The model under review builds one solid part; all positions refer to its coordinate system, in mm. A direction names the side the tool comes from. Coordinates: 2 decimals unless noted, no trailing zeros. Write each loop counter-clockwise with the first axis right and the second up, starting at its lowest first coordinate (ties: lowest second). Pieces come first, ordered by that corner, then holes.
```python
from build123d import *

# Parameters (mm, degrees)
F1_DEPTH = 24
F2_DEPTH = 12


with BuildPart() as f1:
    # F0 (on Front) → F1 (new body)
    with BuildSketch(Plane.XZ):
        Polygon((0, 32), (0, 0), (28.475209, 0), (10, 32), align=None)
        Polygon((10, 32), (28.475209, 0), (39.524791, 0), (58, 32), align=None)
        Polygon((58, 32), (39.524791, 0), (68, 0), (68, 32), align=None)
    extrude(amount=-F1_DEPTH)

    # F0 (on Front) → F2 (cut)
    with BuildSketch(Plane.XZ):
        Polygon((10, 32), (28.475209, 0), (39.524791, 0), (58, 32), align=None)
    extrude(amount=-F2_DEPTH, mode=Mode.SUBTRACT)


solid = f1.part
```
Item 1: Take a section at B-B, the plane z = 13.5. Write out the cut boundary in (x, y).
Solved:
outline: (0, 0) - (20.68, 0) - (20.68, 12) - (47.32, 12) - (47.32, 0) - (68, 0) - (68, 24) - (0, 24) - close
Item 2: For pin 1 (1 mm diameter, centred on x = 29.5, y = 6.5, fed in from +Z); pin 2 (6 mm diameter, centred on x = 16, y = 5.5, fed in from +Z), all flat-tipped, find the tip position at first contact; note any pin that passes through.
Solved:
pin 1: passes through
pin 2: stops at z = 26.8
Item 3: Take a section at A-A, the plane y = 7. Write out the cut boundary in (x, z).
Solved:
outline: (0, 0) - (28.48, 0) - (10, 32) - (0, 32) - close; (39.52, 0) - (68, 0) - (68, 32) - (58, 32) - close
Item 4: Machinability: for faces 5 (the face through (34, 14, 0)), 6 (the face through (34, 12, 20)), which of the approach directions +Z, -Z, +X, -X, +Y, -Y give a long, thin tool a straight path to every point of the face, cutting with its end or side? Answer none if there is none.
Solved:
face 5: -Z, +X, -X, +Y, -Y
face 6: +Z, -Y
Item 5: Take a section at D-D, the plane z = 7.5. Write out the cut boundary in (x, y).
Solved:
outline: (0, 0) - (24.15, 0) - (24.15, 12) - (43.85, 12) - (43.85, 0) - (68, 0) - (68, 24) - (0, 24) - close
Item 6: Mouldability with a two-part tool opening along X and no side actions: class faces 1 (the face through (19.11, 5.92, 16.22)), 2 (the face through (0, 12, 16)), 3 (the face through (34, 17, 32)), 4 (the face through (48.633, 5.916, 15.776)) as pulls with the +X half, pulls with the -X half, needs draft (parallel to the pull), parting line crosses it, or undercut.
Solved:
face 1: undercut
face 2: pulls with the -X half
face 3: needs draft
face 4: undercut
Item 7: To check wall thickness, follow line 1 along X through (y, z) = (8, 11.5); line 2 along X through (y, z) = (1.75, 16); line 3 along Z through (x, y) = (23, 3). State the ranges of each line that lie inside material, in increasing order.
Solved:
line 1: x = 0 to 21.84, 46.16 to 68
line 2: x = 0 to 19.24, 48.76 to 68
line 3: z = 0 to 9.48
Item 8: Take a section at C-C, the plane x = 26. Write out the cut boundary in (y, z), plus the area to 3 significant figures.
Solved:
outline: (0, 0) - (24, 0) - (24, 32) - (12, 32) - (12, 4.29) - (0, 4.29) - close
area: 435 mm2
